from build123d import *

# Parameters (mm, degrees)
F0_R      = 18.4
F1_DEPTH  = 22
F2_R      = 17.25
F3_DEPTH  = 30.7
F4_R      = 6
F5_DEPTH  = 6.5
F6_R      = 3
F7_DEPTH  = 15.5
F8_SIZE   = 1
F10_DEPTH = 12
F12_D     = 3
F12_DEPTH = 24
F12_TIP   = 0.9012909285
F14_DEPTH = 1
F15_R     = 6.5
F16_DEPTH = 1.5
F17_SIZE  = 1
F18_W     = 3.175
F18_H     = 0.79375
F19_DEPTH = 5.6
F20_SIZE  = 1
F22_DEPTH = 25.4
F23_R     = 0.5
F24_R     = 17
F25_DEPTH = 15.4


with BuildPart() as f1:
    # F0 (on Front) → F1 (new body)
    with BuildSketch(Plane.XZ):
        Circle(F0_R)
    extrude(amount=F1_DEPTH)

    # F2 (on face) → F3 (join)
    with BuildSketch(Plane(origin=(0, 0, 0), x_dir=(-1, 0, 0), z_dir=(0, 1, 0))):
        Circle(F2_R)
    extrude(amount=F3_DEPTH)

    # F4 (on face) → F5 (join)
    with BuildSketch(Plane.XZ.offset(22)):
        with Locations((7, 0)):
            Circle(F4_R)
    extrude(amount=F5_DEPTH)

    # F6 (on face) → F7 (join)
    with BuildSketch(Plane.XZ.offset(28.5)):
        with Locations((7, 0)):
            Circle(F6_R)
    extrude(amount=F7_DEPTH)

    # F8
    f8_edges = [f1.edges().sort_by_distance(p)[0] for p in [
        (1, -28.5, 0),
    ]]
    chamfer(f8_edges, length=F8_SIZE)

    # F9 (on face) → F10 (cut)
    with BuildSketch(Plane.XZ.offset(44)):
        with BuildLine():
            ThreePointArc((8.8, 2.4), (7, 3), (5.2, 2.4))
            Line((5.2, 2.4), (8.8, 2.4))
        make_face()
    extrude(amount=-F10_DEPTH, mode=Mode.SUBTRACT)

    # F12
    with Locations(Plane.XZ.offset(22)):
        with Locations((0, 15.5), (-13.4233937587, 7.75), (-13.4233937587, -7.75), (0, -15.5), (13.4233937587, -7.75), (13.4233937587, 7.75)):
            Hole(F12_D / 2, depth=F12_DEPTH)
            with Locations((0, 0, -(F12_DEPTH + F12_TIP / 2))):  # 118° drill point
                Cone(0, F12_D / 2, F12_TIP, mode=Mode.SUBTRACT)

    # F13 (on face) → F14 (cut)
    with BuildSketch(Plane.XZ.offset(22)):
        with BuildLine():
            ThreePointArc((7.1428571429, 7.9987243881), (8.1017881451, 8.6603638261), (7.7833850932, 9.7810488441))
            ThreePointArc((7.7833850932, 9.7810488441), (-12.5, 0), (7.7833850932, -9.7810488441))
            ThreePointArc((7.7833850932, -9.7810488441), (8.1017881451, -8.6603638261), (7.1428571429, -7.9987243881))
            ThreePointArc((7.1428571429, -7.9987243881), (-1, 0), (7.1428571429, 7.9987243881))
        make_face()
    extrude(amount=-F14_DEPTH, mode=Mode.SUBTRACT)

    # F15 (on face) → F16 (join)
    with BuildSketch(Plane(origin=(0, 30.7, 0), x_dir=(-1, 0, 0), z_dir=(0, 1, 0))):
        Circle(F15_R)
    extrude(amount=F16_DEPTH)

    # F17
    f17_edges = [f1.edges().sort_by_distance(p)[0] for p in [
        (6.5, 32.2, 0),
    ]]
    chamfer(f17_edges, length=F17_SIZE)

    # F18 (on face) → F19 (join)
    with BuildSketch(Plane(origin=(0, 30.7, 0), x_dir=(-1, 0, 0), z_dir=(0, 1, 0))):
        with Locations((0, 11.653125)):
            Rectangle(F18_W, F18_H)
        with Locations((0, -11.653125)):
            Rectangle(F18_W, F18_H)
    extrude(amount=F19_DEPTH)

    # F20
    f20_edges = [f1.edges().sort_by_distance(p)[0] for p in [
        (-1.5875, 36.3, 11.653125),
        (1.5875, 36.3, 11.653125),
        (1.5875, 36.3, -11.653125),
        (-1.5875, 36.3, -11.653125),
    ]]
    chamfer(f20_edges, length=F20_SIZE)

    # F21 (on face) → F22 (cut)
    with BuildSketch(Plane.XY.offset(12.05)):
        with BuildLine():
            Line((0.5, 33.74), (0.5, 35.01))
            ThreePointArc((0.5, 35.01), (0, 35.51), (-0.5, 35.01))
            Line((-0.5, 35.01), (-0.5, 33.74))
            ThreePointArc((-0.5, 33.74), (0, 33.24), (0.5, 33.74))
        make_face()
    extrude(amount=-F22_DEPTH, mode=Mode.SUBTRACT)

    # F23
    f23_edges = [f1.edges().sort_by_distance(p)[0] for p in [
        (-18.4, -22, 0),
    ]]
    fillet(f23_edges, radius=F23_R)

    # F24 (on face) → F25 (join)
    with BuildSketch(Plane(origin=(0, 30.7, 0), x_dir=(-1, 0, 0), z_dir=(0, 1, 0))):
        Circle(F24_R)
    extrude(amount=F25_DEPTH)


solid = f1.part
For this review, take the finished solid that the model builds, in its own axes (mm). A direction names the side the tool comes from. Coordinates: 2 decimals unless noted, no trailing zeros. Loops run counter-clockwise (first coordinate to the right, second up) from the corner with the lowest first, then second, coordinate; pieces in that order, holes last. Notation, with made-up numbers: (87, 65) - (145, 65) arc R15 ccw to (145, 69) - close; hole circle Ø6 at (44.5, 22). An arc over 180 degrees is marked (long way). Return JSON: item names as keys, results as strings.
Item 1: Insertion check: pin 1 (20 mm diameter, centred on x = 0, z = 0, fed in from -Y); pin 2 (1.8 mm diameter, centred on x = 7, y = -37, fed in from +Z); pin 3 (1 mm diameter, centred on x = 12, z = -6.5, fed in from -Y); pin 4 (10.5 mm diameter, centred on x = -1, z = 5.5, fed in from -Y). Each pin has a flat end and moves straight along its axis. Give the tip position at first contact, or say it passes through.
Determined:
{"pin 1": "stops at y = -44", "pin 2": "stops at z = 2.4", "pin 3": "stops at y = -22", "pin 4": "stops at y = -28.5"}
Item 2: Take a section at A-A (y = -3.5). Give the boundary of the cut face in (x, z).
Determined:
{"outline": "circle Ø36.8 at (0, 0); hole circle Ø3 at (-13.42, -7.75); hole circle Ø3 at (-13.42, 7.75); hole circle Ø3 at (0, -15.5); hole circle Ø3 at (0, 15.5); hole circle Ø3 at (13.42, -7.75); hole circle Ø3 at (13.42, 7.75)"}
Item 3: Mouldability with a two-part tool opening along Z and no side actions: class faces 3 (the cylindrical face through (1, -25, 0)), 4 (the conical face through (13.664, 2.745, -7.85)), 5 (the flat face through (0, 46.1, 0)) as pulls with the +Z half, pulls with the -Z half, needs draft (parallel to the pull), parting line crosses it, or undercut.
Determined:
{"face 3": "parting line crosses it", "face 4": "undercut", "face 5": "needs draft"}
Item 4: Take a section at C-C (y = 40). Give the boundary of the cut face in (x, z).
Determined:
{"outline": "circle Ø34 at (0, 0)"}
Item 5: For line 1 (Z direction, x = 0, y = -8); line 2 (Z direction, x = 0, y = -21.45); line 3 (Z direction, x = 1, y = -18), list the stretches that pass through material, from the lowest coordinate up.
Determined:
{"line 1": "z = -18.4 to -17, -14 to 14, 17 to 18.4", "line 2": "z = -18.4 to -17, -14 to -12.5, -3.87 to 3.87, 12.5 to 14, 17 to 18.4", "line 3": "z = -18.37 to -16.62, -14.38 to 14.38, 16.62 to 18.37"}
Item 6: Take a section at B-B (z = 0). Give the boundary of the cut face in (x, y).
Determined:
{"outline": "(-18.4, -21.5) arc R0.5 ccw to (-17.9, -22) - (-12.5, -22) - (-12.5, -21) - (-1, -21) - (-1, -22) - (1, -22) - (1, -27.5) - (2, -28.5) - (4, -28.5) - (4, -44) - (10, -44) - (10, -28.5) - (12, -28.5) - (13, -27.5) - (13, -22) - (17.9, -22) arc R0.5 ccw to (18.4, -21.5) - (18.4, 0) - (17.25, 0) - (17.25, 30.7) - (17, 30.7) - (17, 46.1) - (-17, 46.1) - (-17, 30.7) - (-17.25, 30.7) - (-17.25, 0) - (-18.4, 0) - close"}
Item 7: For faces 1 (the cylindrical face through (-14.6, -10.6, -11.2)), 2 (the cylindrical face through (-14.81, -9.83, -8.32)), list the 3-axis set-ups (+Z, -Z, +X, -X, +Y, -Y) from which the entire face can be reached by the end or side of a thin tool; tool diameter is ignored.
Determined:
{"face 1": "+Y, -Y", "face 2": "-Y"}
